For this review, use the dimensioned drawing (mm, ordinates from the lowest corner) and the shaded views. Give positions to 0.01 mm unless a question says otherwise; leave off trailing zeros. Loops run counter-clockwise (first coordinate to the right, second up) from the corner with the lowest first, then second, coordinate; pieces in that order, holes last. Notation, with made-up numbers: M 8,84.25 L 14,84.25 A15 ccw 14,109.25 Z; hole C -21.5,-35.5 d6. An arc over 180 degrees is marked long. Return JSON: item names as keys, results as strings.
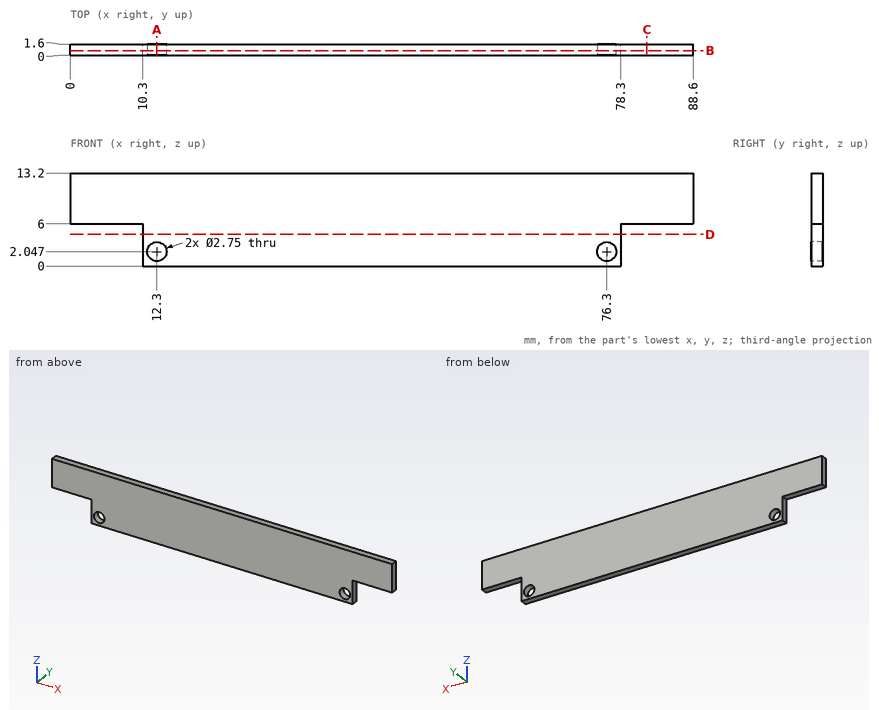
1) Consider section D-D on z = 4.5. Write out the cut boundary in (x, y), then the cut area to 3 significant figures.
From the geometry:
{"outline": "M 10.3,0 L 78.3,0 L 78.3,1.6 L 10.3,1.6 Z", "area": "109 mm²"}
2) Consider section A-A on x = 12.3. Write out the cut boundary in (y, z), then the cut area to 3 significant figures.
From the geometry:
{"outline": "M 0,0 L 1.6,0 L 1.6,0.67 L 0,0.67 Z; M 0,3.42 L 1.6,3.42 L 1.6,13.2 L 0,13.2 Z", "area": "16.7 mm²"}
3) Consider section C-C on x = 82. Write out the cut boundary in (y, z), then the cut area to 3 significant figures.
From the geometry:
{"outline": "M 0,6 L 1.6,6 L 1.6,13.2 L 0,13.2 Z", "area": "11.5 mm²"}
4) Insertion check: pin 1 (3.5 mm diameter, centred on x = 76.3, z = 2.05, fed in from +Y); pin 2 (0.5 mm diameter, centred on y = 1, z = 3.5, fed in from +X). Each pin has a flat end and moves straight along its axis. Give the tip position at first contact, or say it passes through.
From the geometry:
{"pin 1": "y = 1.6", "pin 2": "x = 78.3"}
5) Wall thickness on L1, parallel to Z at x = 76.3, y = 0.95; L2, parallel to X at y = 1.4, z = 4.25: over which ranges is each line inside the solid? List them lowest first. Write a range as from..to.
From the geometry:
{"L1": "0..0.67, 3.42..13.2", "L2": "10.3..78.3"}
6) Consider section B-B on y = 0.65. Count the separate pieces of the cut face and the enclosed holes in it, then the cut area to 3 significant figures.
From the geometry:
{"separate pieces": "1", "enclosed holes": "2", "area": "1,030 mm²"}
